Part model, mm, in its own coordinate system. Face numbers are marked on the shaded views. Coordinates: 2 decimals unless noted, no trailing zeros. Write each loop counter-clockwise with the first axis right and the second up, starting at its lowest first coordinate (ties: lowest second). Pieces come first, ordered by that corner, then holes. Notation, with made-up numbers: (28, 23) -> (66, 23) arc R22 cw to (66, 62) -> close; hole circle Ø1 at (-38, -10). An arc over 180 degrees is marked (long way). One line per question, with ' | ' between items. Start each with the question number.
Item 1: Saw through at B-B (x = -95.5). List the corners of the cut face in (y, z), and give its area (3 significant figures).
Item 2: Two-plate mould, pull along Y, no slides. Class the marked faces 1 and 2: pulls with the +Y half, pulls with the -Y half, needs draft (parallel to the pull), parting line crosses it, or undercut.
Item 3: Pin check, flat tips, straight feed: pin 1 (6 mm diameter, centred on x = -102.5, y = 14.5, fed in from +Z); pin 2 (1.5 mm diameter, centred on x = -87, z = 30, fed in from +Y); pin 3 (2 mm diameter, centred on x = -107.5, z = 37, fed in from -Y). Stop position of each tip, or through.
Item 4: Saw through at A-A (y = 19.5). List the corners of the cut face in (x, z).
Item 5: Saw through at D-D (y = 16.75). List the corners of the cut face in (x, z).
Item 6: Saw through at C-C (y = 9.5). List the corners of the cut face in (x, z), and give its area (3 significant figures).
Item 7: Probe probe 1 along X at (y, z) = (14.75, 28); probe 2 along Y at (x, z) = (-86.75, 32.5); probe 3 along Y at (x, z) = (-86.25, 32). List the from-to ranges inside material, lowest first. Write a range as [from, to].
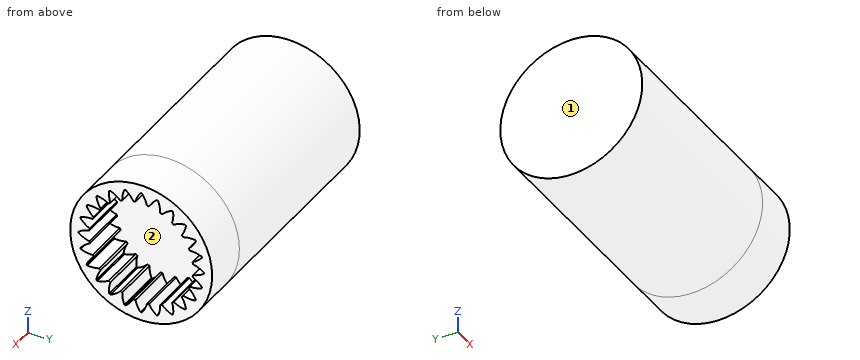
from build123d import *

# Parameters (mm, degrees)
INTERNAL_START                  = -88.407440494
INTERNAL_SPUR_GEAR_AM_OUTLINE_R = 7.5
INTERNAL_SPUR_GEAR_AM_DEPTH     = 5
BOSS_EXTRUDE2_START             = 22.1
SKETCH3_R                       = 7.5
BOSS_EXTRUDE2_DEPTH             = 22.1


# Read off the part's stored shape, not the designer's step: internal spur gear_am
with BuildPart() as part:
    # internal spur gear_am outline → internal spur gear_am (new body)
    with BuildSketch(Plane.YZ.offset(INTERNAL_START)):
        with Locations((15.590226083, 31.241752714)):
            Circle(INTERNAL_SPUR_GEAR_AM_OUTLINE_R)
        with BuildLine():
            ThreePointArc((22.215876043, 31.173645397), (21.665278496, 30.84231879), (21.056750139, 30.635852768))
            ThreePointArc((21.056750139, 30.635852768), (21.043172821, 30.523858657), (21.027301295, 30.412166585))
            ThreePointArc((21.027301295, 30.412166585), (21.561657212, 30.055236993), (22.007739967, 29.592694935))
            ThreePointArc((22.007739967, 29.592694935), (21.990450608, 29.526817722), (21.972485025, 29.461121702))
            ThreePointArc((21.972485025, 29.461121702), (21.354894998, 29.283589907), (20.713664403, 29.241657772))
            ThreePointArc((20.713664403, 29.241657772), (20.671563512, 29.136993836), (20.62732476, 29.033215432))
            ThreePointArc((20.62732476, 29.033215432), (21.051092764, 28.550146434), (21.362260924, 27.987910402))
            ThreePointArc((21.362260924, 27.987910402), (21.328510409, 27.928752714), (21.294153607, 27.869945067))
            ThreePointArc((21.294153607, 27.869945067), (20.65165884, 27.858306583), (20.021424813, 27.98376594))
            ThreePointArc((20.021424813, 27.98376594), (19.953669455, 27.893564855), (19.884078274, 27.804772446))
            ThreePointArc((19.884078274, 27.804772446), (20.168379277, 27.228484394), (20.323427246, 26.604869844))
            ThreePointArc((20.323427246, 26.604869844), (20.275515615, 26.556463182), (20.227108954, 26.508551552))
            ThreePointArc((20.227108954, 26.508551552), (19.603494404, 26.663599521), (19.027206352, 26.947900524))
            ThreePointArc((19.027206352, 26.947900524), (18.938413943, 26.878309343), (18.848212857, 26.810553985))
            ThreePointArc((18.848212857, 26.810553985), (18.973672215, 26.180319958), (18.96203373, 25.537825191))
            ThreePointArc((18.96203373, 25.537825191), (18.903226083, 25.503468389), (18.844068396, 25.469717874))
            ThreePointArc((18.844068396, 25.469717874), (18.281832364, 25.780886034), (17.798763365, 26.204654038))
            ThreePointArc((17.798763365, 26.204654038), (17.694984961, 26.160415286), (17.590321026, 26.118314394))
            ThreePointArc((17.590321026, 26.118314394), (17.548388891, 25.4770838), (17.370857096, 24.859493773))
            ThreePointArc((17.370857096, 24.859493773), (17.305161076, 24.841528189), (17.239283862, 24.824238831))
            ThreePointArc((17.239283862, 24.824238831), (16.776741804, 25.270321586), (16.419812213, 25.804677503))
            ThreePointArc((16.419812213, 25.804677503), (16.308120141, 25.788805977), (16.19612603, 25.775228658))
            ThreePointArc((16.19612603, 25.775228658), (15.989660007, 25.166700302), (15.658333401, 24.616102754))
            ThreePointArc((15.658333401, 24.616102754), (15.590226083, 24.615752714), (15.522118766, 24.616102754))
            ThreePointArc((15.522118766, 24.616102754), (15.190792159, 25.166700301), (14.984326137, 25.775228658))
            ThreePointArc((14.984326137, 25.775228658), (14.872332026, 25.788805977), (14.760639954, 25.804677503))
            ThreePointArc((14.760639954, 25.804677503), (14.403710362, 25.270321586), (13.941168304, 24.824238831))
            ThreePointArc((13.941168304, 24.824238831), (13.87529109, 24.841528189), (13.809595071, 24.859493773))
            ThreePointArc((13.809595071, 24.859493773), (13.632063276, 25.4770838), (13.59013114, 26.118314394))
            ThreePointArc((13.59013114, 26.118314394), (13.485467205, 26.160415286), (13.381688801, 26.204654038))
            ThreePointArc((13.381688801, 26.204654038), (12.898619802, 25.780886034), (12.33638377, 25.469717874))
            ThreePointArc((12.33638377, 25.469717874), (12.277226083, 25.503468389), (12.218418436, 25.537825191))
            ThreePointArc((12.218418436, 25.537825191), (12.206779952, 26.180319958), (12.332239309, 26.810553985))
            ThreePointArc((12.332239309, 26.810553985), (12.242038224, 26.878309343), (12.153245815, 26.947900524))
            ThreePointArc((12.153245815, 26.947900524), (11.576957763, 26.663599521), (10.953343213, 26.508551552))
            ThreePointArc((10.953343213, 26.508551552), (10.904936551, 26.556463182), (10.857024921, 26.604869844))
            ThreePointArc((10.857024921, 26.604869844), (11.01207289, 27.228484394), (11.296373893, 27.804772446))
            ThreePointArc((11.296373893, 27.804772446), (11.226782712, 27.893564855), (11.159027354, 27.98376594))
            ThreePointArc((11.159027354, 27.98376594), (10.528793327, 27.858306583), (9.88629856, 27.869945067))
            ThreePointArc((9.88629856, 27.869945067), (9.851941758, 27.928752714), (9.818191243, 27.987910402))
            ThreePointArc((9.818191243, 27.987910402), (10.129359403, 28.550146434), (10.553127407, 29.033215432))
            ThreePointArc((10.553127407, 29.033215432), (10.508888654, 29.136993836), (10.466787763, 29.241657772))
            ThreePointArc((10.466787763, 29.241657772), (9.825557169, 29.283589907), (9.207967142, 29.461121702))
            ThreePointArc((9.207967142, 29.461121702), (9.190001558, 29.526817721), (9.1727122, 29.592694935))
            ThreePointArc((9.1727122, 29.592694935), (9.618794955, 30.055236993), (10.153150872, 30.412166585))
            ThreePointArc((10.153150872, 30.412166585), (10.137279346, 30.523858657), (10.123702027, 30.635852768))
            ThreePointArc((10.123702027, 30.635852768), (9.51517367, 30.84231879), (8.964576123, 31.173645397))
            ThreePointArc((8.964576123, 31.173645397), (8.964226083, 31.241752715), (8.964576123, 31.309860032))
            ThreePointArc((8.964576123, 31.309860032), (9.51517367, 31.641186639), (10.123702027, 31.847652661))
            ThreePointArc((10.123702027, 31.847652661), (10.137279346, 31.959646772), (10.153150872, 32.071338844))
            ThreePointArc((10.153150872, 32.071338844), (9.618794955, 32.428268436), (9.1727122, 32.890810493))
            ThreePointArc((9.1727122, 32.890810493), (9.190001558, 32.956687707), (9.207967142, 33.022383727))
            ThreePointArc((9.207967142, 33.022383727), (9.825557169, 33.199915522), (10.466787763, 33.241847657))
            ThreePointArc((10.466787763, 33.241847657), (10.508888654, 33.346511592), (10.553127407, 33.450289996))
            ThreePointArc((10.553127407, 33.450289996), (10.129359403, 33.933358995), (9.818191243, 34.495595027))
            ThreePointArc((9.818191243, 34.495595027), (9.851941758, 34.554752714), (9.88629856, 34.613560362))
            ThreePointArc((9.88629856, 34.613560362), (10.528793327, 34.625198846), (11.159027354, 34.499739488))
            ThreePointArc((11.159027354, 34.499739488), (11.226782712, 34.589940574), (11.296373893, 34.678732983))
            ThreePointArc((11.296373893, 34.678732983), (11.01207289, 35.255021035), (10.857024921, 35.878635585))
            ThreePointArc((10.857024921, 35.878635585), (10.904936551, 35.927042247), (10.953343213, 35.974953877))
            ThreePointArc((10.953343213, 35.974953877), (11.576957763, 35.819905908), (12.153245815, 35.535604905))
            ThreePointArc((12.153245815, 35.535604905), (12.242038224, 35.605196086), (12.332239309, 35.672951444))
            ThreePointArc((12.332239309, 35.672951444), (12.206779952, 36.303185471), (12.218418436, 36.945680238))
            ThreePointArc((12.218418436, 36.945680238), (12.277226083, 36.98003704), (12.33638377, 37.013787555))
            ThreePointArc((12.33638377, 37.013787555), (12.898619802, 36.702619395), (13.381688801, 36.278851391))
            ThreePointArc((13.381688801, 36.278851391), (13.485467205, 36.323090143), (13.59013114, 36.365191035))
            ThreePointArc((13.59013114, 36.365191035), (13.632063276, 37.006421629), (13.809595071, 37.624011656))
            ThreePointArc((13.809595071, 37.624011656), (13.875291091, 37.641977239), (13.941168304, 37.659266598))
            ThreePointArc((13.941168304, 37.659266598), (14.403710362, 37.213183843), (14.760639954, 36.678827926))
            ThreePointArc((14.760639954, 36.678827926), (14.872332026, 36.694699452), (14.984326137, 36.70827677))
            ThreePointArc((14.984326137, 36.70827677), (15.190792159, 37.316805127), (15.522118766, 37.867402675))
            ThreePointArc((15.522118766, 37.867402675), (15.590226084, 37.867752714), (15.658333401, 37.867402675))
            ThreePointArc((15.658333401, 37.867402675), (15.989660007, 37.316805127), (16.19612603, 36.70827677))
            ThreePointArc((16.19612603, 36.70827677), (16.308120141, 36.694699452), (16.419812213, 36.678827926))
            ThreePointArc((16.419812213, 36.678827926), (16.776741804, 37.213183843), (17.239283862, 37.659266598))
            ThreePointArc((17.239283862, 37.659266598), (17.305161076, 37.641977239), (17.370857096, 37.624011656))
            ThreePointArc((17.370857096, 37.624011656), (17.548388891, 37.006421629), (17.590321026, 36.365191035))
            ThreePointArc((17.590321026, 36.365191035), (17.694984961, 36.323090143), (17.798763365, 36.278851391))
            ThreePointArc((17.798763365, 36.278851391), (18.281832364, 36.702619395), (18.844068396, 37.013787555))
            ThreePointArc((18.844068396, 37.013787555), (18.903226083, 36.98003704), (18.96203373, 36.945680238))
            ThreePointArc((18.96203373, 36.945680238), (18.973672215, 36.303185471), (18.848212857, 35.672951444))
            ThreePointArc((18.848212857, 35.672951444), (18.938413943, 35.605196086), (19.027206352, 35.535604905))
            ThreePointArc((19.027206352, 35.535604905), (19.603494404, 35.819905908), (20.227108954, 35.974953877))
            ThreePointArc((20.227108954, 35.974953877), (20.275515616, 35.927042247), (20.323427246, 35.878635585))
            ThreePointArc((20.323427246, 35.878635585), (20.168379277, 35.255021035), (19.884078274, 34.678732983))
            ThreePointArc((19.884078274, 34.678732983), (19.953669455, 34.589940574), (20.021424813, 34.499739488))
            ThreePointArc((20.021424813, 34.499739488), (20.65165884, 34.625198846), (21.294153607, 34.613560362))
            ThreePointArc((21.294153607, 34.613560362), (21.328510409, 34.554752714), (21.362260924, 34.495595027))
            ThreePointArc((21.362260924, 34.495595027), (21.051092764, 33.933358995), (20.62732476, 33.450289996))
            ThreePointArc((20.62732476, 33.450289996), (20.671563512, 33.346511592), (20.713664403, 33.241847657))
            ThreePointArc((20.713664403, 33.241847657), (21.354894998, 33.199915522), (21.972485025, 33.022383727))
            ThreePointArc((21.972485025, 33.022383727), (21.990450608, 32.956687707), (22.007739967, 32.890810493))
            ThreePointArc((22.007739967, 32.890810493), (21.561657212, 32.428268436), (21.027301295, 32.071338844))
            ThreePointArc((21.027301295, 32.071338844), (21.043172821, 31.959646772), (21.056750139, 31.847652661))
            ThreePointArc((21.056750139, 31.847652661), (21.665278496, 31.641186639), (22.215876043, 31.309860032))
            ThreePointArc((22.215876043, 31.309860032), (22.216226083, 31.241752714), (22.215876043, 31.173645397))
        make_face(mode=Mode.SUBTRACT)
    extrude(amount=INTERNAL_SPUR_GEAR_AM_DEPTH)

    # Sketch3 → Boss-Extrude2 (add)
    with BuildSketch(Plane.ZY.offset(88.407440494).offset(BOSS_EXTRUDE2_START)):
        with Locations((31.241752714, 15.590226083)):
            Circle(SKETCH3_R)
    extrude(amount=-BOSS_EXTRUDE2_DEPTH)


solid = part.part
From the geometry:
1) outline: circle Ø15 at (15.59, 31.24) | area: 177 mm2
2) face 1: needs draft | face 2: undercut
3) pin 1: z = 38.74 | pin 2: y = 23.07 | pin 3: y = 9.79
4) outline: (-110.51, 24.84) -> (-83.41, 24.84) -> (-83.41, 26.7) -> (-88.41, 26.7) -> (-88.41, 35.78) -> (-83.41, 35.78) -> (-83.41, 37.64) -> (-110.51, 37.64) -> close
5) outline: (-110.51, 23.83) -> (-83.41, 23.83) -> (-83.41, 25.3) -> (-88.41, 25.3) -> (-88.41, 37.18) -> (-83.41, 37.18) -> (-83.41, 38.65) -> (-110.51, 38.65) -> close
6) outline: (-110.51, 26.86) -> (-83.41, 26.86) -> (-83.41, 29.36) -> (-88.41, 29.36) -> (-88.41, 29.95) -> (-83.41, 29.95) -> (-83.41, 30.85) -> (-88.41, 30.85) -> (-88.41, 31.63) -> (-83.41, 31.63) -> (-83.41, 32.53) -> (-88.41, 32.53) -> (-88.41, 33.12) -> (-83.41, 33.12) -> (-83.41, 35.62) -> (-110.51, 35.62) -> close | area: 227 mm2
7) probe 1: [-110.51, -88.41] | probe 2: [8.2, 9.54], [21.64, 22.98] | probe 3: [8.13, 10.14], [21.04, 23.05]
